Source: three-view drawing plus pictorial views. Frame: mm from the lowest corner of the part. A direction names the side the tool comes from. Round coordinates to 2 decimals unless told otherwise and drop trailing zeros. Write each loop counter-clockwise with the first axis right and the second up, starting at its lowest first coordinate (ties: lowest second). Pieces come first, ordered by that corner, then holes. Notation, with made-up numbers: (60.5, 36.25) - (73.5, 36.25) arc R14 ccw to (73.5, 57.25) - close; hole circle Ø6 at (-31.5, -30.5). An arc over 180 degrees is marked (long way). Write each question's results on one line, items separated by ' | '.
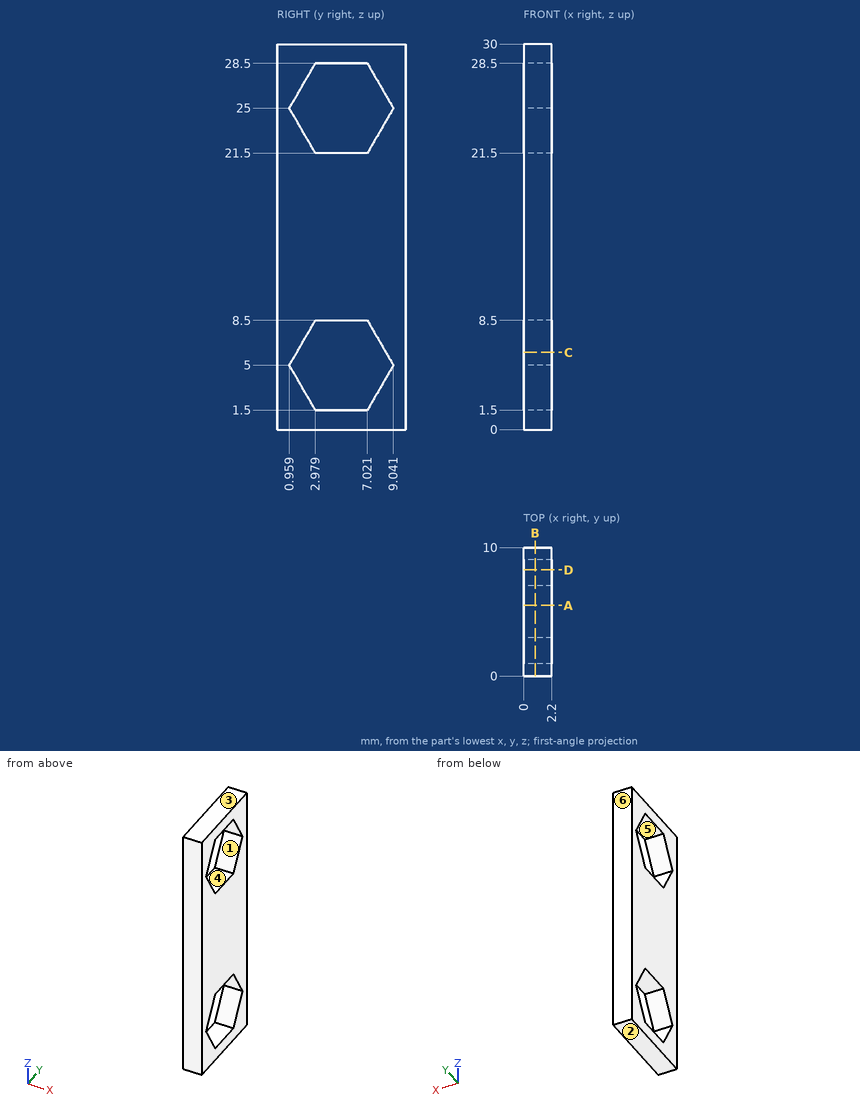
Q1. Mould query, pull axis Y, two halves, no side actions, for the marked faces 3, 4, 5 and 6. Classes: pulls with the +Y half, pulls with the -Y half, needs draft (parallel to the pull), parting line crosses it, or undercut.
Answer block:
face 3: needs draft | face 4: undercut | face 5: undercut | face 6: pulls with the +Y half
Q2. Section query C-C, the plane z = 6. Return loops of the section in (x, y) (1 decimal).
Answer block:
outline: (0, 0) - (2.2, 0) - (2.2, 1.5) - (0, 1.5) - close; (0, 8.5) - (2.2, 8.5) - (2.2, 10) - (0, 10) - close
Q3. Section query B-B, the plane x = 0.9. Return loops of the section in (y, z), plus the area to 3 significant figures.
Answer block:
outline: (0, 0) - (10, 0) - (10, 30) - (0, 30) - close; hole (0.96, 5) - (2.98, 1.5) - (7.02, 1.5) - (9.04, 5) - (7.02, 8.5) - (2.98, 8.5) - close; hole (0.96, 25) - (2.98, 21.5) - (7.02, 21.5) - (9.04, 25) - (7.02, 28.5) - (2.98, 28.5) - close | area: 215 mm2
Q4. Section query A-A, the plane y = 5.5. Return loops of the section in (x, z), plus the area to 3 significant figures.
Answer block:
outline: (0, 0) - (2.2, 0) - (2.2, 1.5) - (0, 1.5) - close; (0, 8.5) - (2.2, 8.5) - (2.2, 21.5) - (0, 21.5) - close; (0, 28.5) - (2.2, 28.5) - (2.2, 30) - (0, 30) - close | area: 35.2 mm2
Q5. Access query for the marked faces 1 and 2. Directions: +Z, -Z, +X, -X, +Y, -Y. A direction counts if a zero-diameter tool reaches every point of the face in a straight line with its end or side. Return the directions, or none.
Answer block:
face 1: +X, -X | face 2: -Z, +X, -X, +Y, -Y
Q6. Pin query (flat end, axial travel): pin 1 (0.7 mm diameter, centred on x = 1, y = 5.5, fed in from -Z); pin 2 (1 mm diameter, centred on y = 5, z = 7.5, fed in from -X). Return the tip coordinate at first contact, or that it passes through.
Answer block:
pin 1: z = 0 | pin 2: through
Q7. Ray query, line 1 along Z through (x, y) = (0.7, 4.75); line 2 along Z through (x, y) = (0.4, 1.25) (1 decimal); line 3 along Y through (x, z) = (0.6, 6.5) (1 decimal). Return the intervals inside material, ascending.
Answer block:
line 1: 0 to 1.5, 8.5 to 21.5, 28.5 to 30 | line 2: 0 to 4.5, 5.5 to 24.5, 25.5 to 30 | line 3: 0 to 1.8, 8.2 to 10
Q8. Section query D-D, the plane y = 8.25. Return loops of the section in (x, z).
Answer block:
outline: (0, 0) - (2.2, 0) - (2.2, 3.63) - (0, 3.63) - close; (0, 6.37) - (2.2, 6.37) - (2.2, 23.63) - (0, 23.63) - close; (0, 26.37) - (2.2, 26.37) - (2.2, 30) - (0, 30) - close
